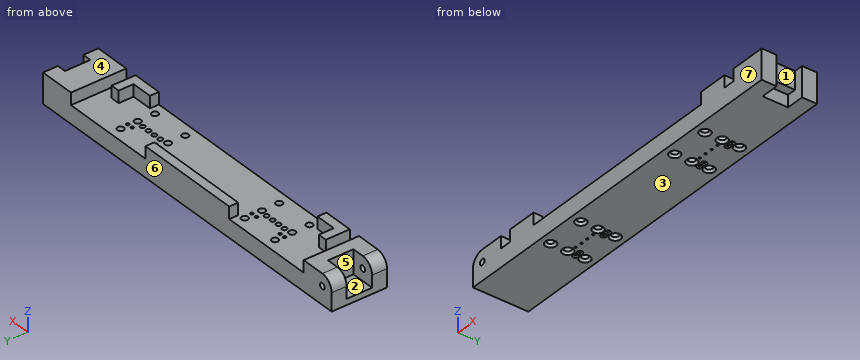
from build123d import *

# Parameters (mm, degrees)
SKETCH_W         = 124
SKETCH_H         = 18.5
SKETCH_R         = 0.5
PAD_DEPTH        = 6
HOLE_D           = 0.7
HOLE_DEPTH       = 25
HOLE_CBORE_D     = 1.6
HOLE_CBORE_DEPTH = 2.1
CHAMFER_SIZE     = 0.2
SKETCH002_W      = 12
SKETCH002_H      = 18.5
SKETCH002_W_2    = 36
SKETCH002_H_2    = 3
PAD001_DEPTH     = 4
CHAMFER001_SIZE  = 0.4
SKETCH003_R      = 1.1
POCKET_DEPTH     = 10.001
CHAMFER002_SIZE  = 0.7
SKETCH004_W      = 8
SKETCH004_H      = 8.5
POCKET001_DEPTH  = 8
SKETCH005_W      = 8.5
SKETCH005_H      = 4
POCKET002_DEPTH  = 6
SKETCH008_R      = 1
HOLE001_DEPTH    = 18.501
FILLET_R         = 4
SKETCH011_W      = 8.5
SKETCH011_H      = 6
POCKET003_DEPTH  = 3


with BuildPart() as part:
    # Sketch → Pad (new body)
    with BuildSketch(Plane(origin=(0, 0, 0), x_dir=(-1, 0, 0), z_dir=(0, 0, -1))):
        with Locations((0, -6.75)):
            Rectangle(SKETCH_W, SKETCH_H)
        with Locations((-33.67, -3.81)):
            Circle(SKETCH_R, mode=Mode.SUBTRACT)
        with Locations((-31.745, -3.81)):
            Circle(SKETCH_R, mode=Mode.SUBTRACT)
        with Locations((-21.595, -3.81)):
            Circle(SKETCH_R, mode=Mode.SUBTRACT)
        with Locations((-19.67, -3.81)):
            Circle(SKETCH_R, mode=Mode.SUBTRACT)
        with Locations((19.67, -3.81)):
            Circle(SKETCH_R, mode=Mode.SUBTRACT)
        with Locations((21.595, -3.81)):
            Circle(SKETCH_R, mode=Mode.SUBTRACT)
        with Locations((31.745, -3.81)):
            Circle(SKETCH_R, mode=Mode.SUBTRACT)
        with Locations((33.67, -3.81)):
            Circle(SKETCH_R, mode=Mode.SUBTRACT)
    extrude(amount=PAD_DEPTH)

    # Hole
    with Locations(Plane.XY):
        with Locations((-30.48, -6.25), (-27.94, -6.25), (-25.4, -6.25), (-22.86, -6.25), (22.86, -6.25), (25.4, -6.25), (27.94, -6.25), (30.48, -6.25)):
            CounterBoreHole(HOLE_D / 2, HOLE_CBORE_D / 2, HOLE_CBORE_DEPTH, depth=HOLE_DEPTH)

    # Chamfer
    chamfer_edges = [part.edges().sort_by_distance(p)[0] for p in [
        (30.13, -6.25, -2.1),
        (27.59, -6.25, -2.1),
        (25.05, -6.25, -2.1),
        (22.51, -6.25, -2.1),
        (-30.83, -6.25, -2.1),
        (-28.29, -6.25, -2.1),
        (-25.75, -6.25, -2.1),
        (-23.21, -6.25, -2.1),
    ]]
    chamfer(chamfer_edges, length=CHAMFER_SIZE)

    # Sketch002 (on Face25 of Chamfer) → Pad001 (join)
    with BuildSketch(Plane.XY):
        with Locations((-56, -6.75)):
            Rectangle(SKETCH002_W, SKETCH002_H)
        with Locations((56, -6.75)):
            Rectangle(SKETCH002_W, SKETCH002_H)
        with Locations((0, 1)):
            Rectangle(SKETCH002_W_2, SKETCH002_H_2)
        Polygon((-46, -16), (-46, -8), (-43, -8), (-43, -13), (-36, -13), (-36, -16), align=None)
        Polygon((46, -16), (46, -8), (43, -8), (43, -13), (36, -13), (36, -16), align=None)
    extrude(amount=PAD001_DEPTH)

    # Chamfer001
    chamfer001_edges = [part.edges().sort_by_distance(p)[0] for p in [
        (34.17, -3.81, -6),
        (32.245, -3.81, -6),
        (22.095, -3.81, -6),
        (20.17, -3.81, -6),
        (-19.17, -3.81, -6),
        (-21.095, -3.81, -6),
        (-31.245, -3.81, -6),
        (-33.17, -3.81, -6),
    ]]
    chamfer(chamfer001_edges, length=CHAMFER001_SIZE)

    # Sketch003 (on Face23 of Chamfer001) → Pocket (cut, through all)
    with BuildSketch(Plane.XY.offset(4)):
        with Locations((-33.17, -1)):
            Circle(SKETCH003_R)
        with Locations((-20.17, -1)):
            Circle(SKETCH003_R)
        with Locations((-33.17, -6.75)):
            Circle(SKETCH003_R)
        with Locations((-20.17, -6.75)):
            Circle(SKETCH003_R)
        with Locations((-20.17, -12.5)):
            Circle(SKETCH003_R)
        with Locations((-33.17, -12.5)):
            Circle(SKETCH003_R)
        with Locations((20.17, -1)):
            Circle(SKETCH003_R)
        with Locations((33.17, -1)):
            Circle(SKETCH003_R)
        with Locations((20.17, -6.75)):
            Circle(SKETCH003_R)
        with Locations((33.17, -6.75)):
            Circle(SKETCH003_R)
        with Locations((33.17, -12.5)):
            Circle(SKETCH003_R)
        with Locations((20.17, -12.5)):
            Circle(SKETCH003_R)
    extrude(amount=-POCKET_DEPTH, mode=Mode.SUBTRACT)

    # Chamfer002
    chamfer002_edges = [part.edges().sort_by_distance(p)[0] for p in [
        (19.07, -6.75, -6),
        (19.07, -1, -6),
        (19.07, -12.5, -6),
        (32.07, -12.5, -6),
        (32.07, -6.75, -6),
        (32.07, -1, -6),
        (-34.27, -1, -6),
        (-34.27, -6.75, -6),
        (-34.27, -12.5, -6),
        (-21.27, -12.5, -6),
        (-21.27, -6.75, -6),
        (-21.27, -1, -6),
    ]]
    chamfer(chamfer002_edges, length=CHAMFER002_SIZE)

    # Sketch004 (on Face35 of Chamfer002) → Pocket001 (cut)
    with BuildSketch(Plane.XY.offset(4)):
        with Locations((-58, -6.75)):
            Rectangle(SKETCH004_W, SKETCH004_H)
    extrude(amount=-POCKET001_DEPTH, mode=Mode.SUBTRACT)

    # Sketch005 (on Face5 of Pocket001) → Pocket002 (cut)
    with BuildSketch(Plane.YZ.offset(62)):
        with Locations((-6.75, -4)):
            Rectangle(SKETCH005_W, SKETCH005_H)
    extrude(amount=-POCKET002_DEPTH, mode=Mode.SUBTRACT)

    # Sketch008 (on Face3 of Pocket002) → Hole001 (cut, through all)
    with BuildSketch(Plane.XZ.offset(16)):
        with Locations((-58, 0)):
            Circle(SKETCH008_R)
    extrude(amount=-HOLE001_DEPTH, mode=Mode.SUBTRACT)

    # Fillet
    fillet_edges = [part.edges().sort_by_distance(p)[0] for p in [
        (-62, 0, 4),
        (-62, -13.5, 4),
    ]]
    fillet(fillet_edges, radius=FILLET_R)

    # Sketch011 (on Face4 of Pocket002) → Pocket003 (cut)
    with BuildSketch(Plane.YZ.offset(62)):
        with Locations((-6.75, 1)):
            Rectangle(SKETCH011_W, SKETCH011_H)
    extrude(amount=-POCKET003_DEPTH, mode=Mode.SUBTRACT)


solid = part.part
Work out the finished part from the listing and answer in its coordinate system (mm). Face numbers are marked on the shaded views. A direction names the side the tool comes from. Round coordinates to 2 decimals unless told otherwise and drop trailing zeros. Write each loop counter-clockwise with the first axis right and the second up, starting at its lowest first coordinate (ties: lowest second). Pieces come first, ordered by that corner, then holes. Notation, with made-up numbers: (57, -38) - (94, -38) arc R20 ccw to (94, -7) - close; hole circle Ø5 at (26, 30.25). An arc over 180 degrees is marked (long way). Answer in a Markdown table with one row per item. Add a question column.
1. Find the intervals of material crossed by line 1 along X through (y, z) = (1.75, 2.25); line 2 along X through (y, z) = (-8.75, 2.75); line 3 along Y through (x, z) = (25.4, -4.45), in increasing order. Write a range as from..to.
2. Given pin 1 (1.3 mm diameter, centred on x = 28, y = -6, fed in from +Z); pin 2 (1 mm diameter, centred on x = -36.5, z = 1, fed in from +Y); pin 3 (2.5 mm diameter, centred on x = 20.17, y = -12.5, fed in from -Z), each flat-ended and moving along its own axis, determine where each tip first touches the part or whether it passes through.
3. A cutting plane is placed at A-A, the plane x = -10. Determine the outline of the cut face in (y, z), and give its area (3 significant figures).
4. The mould has two halves that part along Y. Classify the marked faces 4, 5, 6 and 7: +Y half, -Y half, draft (parallel to the pull), parting line (faces both ways), or undercut.
5. For the marked faces 1, 2 and 3, determine the directions among +Z, -Z, +X, -X, +Y, -Y from which every point of the face is accessible in a straight line to the end or side of a thin tool.
Worked out:
| question | item | result |
|---|---|---|
| 1 | line 1 | -61.31..-50, -18..18, 50..62 |
| 1 | line 2 | -54..-50, -46..-43, 43..46, 50..59 |
| 1 | line 3 | -16..-6.6, -5.9..2.5 |
| 2 | pin 1 | z = 0 |
| 2 | pin 2 | y = -13 |
| 2 | pin 3 | z = -5.45 |
| 3 | outline | (-16, -6) - (2.5, -6) - (2.5, 4) - (-0.5, 4) - (-0.5, 0) - (-16, 0) - close |
| 3 | area | 123 mm^2 |
| 4 | face 4 | draft |
| 4 | face 5 | undercut |
| 4 | face 6 | +Y half |
| 4 | face 7 | -Y half |
| 5 | face 1 | +Z, -Z, +X |
| 5 | face 2 | +Z, -X |
| 5 | face 3 | -Z, +X, -X, +Y, -Y |
